```python
from build123d import *

# Parameters (mm, degrees)
SKETCH_1_R      = 1.9
SKETCH_1_R_2    = 1
EXTRUDE_1_DEPTH = 16
SKETCH_2_W      = 6
SKETCH_2_H      = 5.8
EXTRUDE_2_DEPTH = 10


with BuildPart() as part:
    # Эскиз1 → Бобышка-Вытянуть1 (new body)
    with BuildSketch(Plane.XY):
        Circle(SKETCH_1_R)
        Circle(SKETCH_1_R_2, mode=Mode.SUBTRACT)
    extrude(amount=EXTRUDE_1_DEPTH)

    # Эскиз2 → Бобышка-Вытянуть2 (add)
    with BuildSketch(Plane.XY):
        with Locations((0, 0.1)):
            Rectangle(SKETCH_2_W, SKETCH_2_H)
    extrude(amount=-EXTRUDE_2_DEPTH)


solid = part.part
```
Verification items for the finished model (mm, model axes). A direction names the side the tool comes from. Coordinates: 2 decimals unless noted, no trailing zeros. Write each loop counter-clockwise with the first axis right and the second up, starting at its lowest first coordinate (ties: lowest second). Pieces come first, ordered by that corner, then holes. Notation, with made-up numbers: (5, 43) - (21, 43) arc R26 ccw to (21, 64) - close; hole circle Ø8 at (82.5, 51.5). An arc over 180 degrees is marked (long way). One line per question, with ' | ' between items. Start each with the question number.
1. Section check D-D (y = 1.3). Enter the section's corners in (x, z), plus the area to 3 significant figures.
2. Draft check along X on faces 1 (the cylindrical face through (0, -1, 8)), 2 (the flat face through (0, 0, 0)), 3 (the flat face through (0, 0, -10)), 4 (the flat face through (-3, 0, -5)). Enter one of: released by +X, released by -X, zero draft, split by the parting line, or undercut.
3. Material ranges on line 1 along Y through (x, z) = (0, 9.5); line 2 along Z through (x, y) = (1.6, 2.5); line 3 along X through (y, z) = (-0.9, 6.25), recorded low to high.
4. Section check C-C (z = 11). Enter the section's corners in (x, y).
5. Gauge pin test, flat ends, axial feed: P1, Ø1.5, axis at x = -2, y = 1, coming from the +Z side; P2, Ø2, axis at x = -0.5, z = 13, coming from the -Y side; P3, Ø3, axis at x = -2, z = 7, coming from the -Y side; P4, Ø0.6, axis at x = 0, y = 0, coming from the +Z side. Record the tip position at first contact, or that the pin passes through.
6. Section check A-A (x = 0). Enter the section's corners in (y, z).
7. Section check B-B (y = 0). Enter the section's corners in (x, z), plus the area to 3 significant figures.
8. Access from +Z, -Z, +X, -X, +Y, -Y to the whole of each face (thin tool, end or side, straight path). Record for faces 5 (the flat face through (0, 2.1, 0)), 6 (the flat face through (0, -2.8, -5)).
Computed values:
1) outline: (-3, -10) - (3, -10) - (3, 0) - (1.39, 0) - (1.39, 16) - (-1.39, 16) - (-1.39, 0) - (-3, 0) - close | area: 104 mm²
2) face 1: undercut | face 2: undercut | face 3: zero draft | face 4: released by -X
3) line 1: -1.9 to -1, 1 to 1.9 | line 2: -10 to 0 | line 3: -1.67 to -0.44, 0.44 to 1.67
4) outline: circle Ø3.8 at (0, 0); hole circle Ø2 at (0, 0)
5) P1: z = 16 | P2: y = -1.9 | P3: y = -1.83 | P4: z = 0
6) outline: (-2.8, -10) - (3, -10) - (3, 0) - (1.9, 0) - (1.9, 16) - (1, 16) - (1, 0) - (-1, 0) - (-1, 16) - (-1.9, 16) - (-1.9, 0) - (-2.8, 0) - close
7) outline: (-3, -10) - (3, -10) - (3, 0) - (1.9, 0) - (1.9, 16) - (1, 16) - (1, 0) - (-1, 0) - (-1, 16) - (-1.9, 16) - (-1.9, 0) - (-3, 0) - close | area: 88.8 mm²
8) face 5: +Z | face 6: +Z, -Z, +X, -X, -Y
